```python
from build123d import *

# Parameters (mm, degrees)
RESSALTO_EXTRUS_O1_DEPTH = 150


with BuildPart() as part:
    # Esboço1 → Ressalto-extrusão1 (new body)
    with BuildSketch(Plane(origin=(0, 0, 0), x_dir=(1, 0, 0), z_dir=(0, 1, 0))):
        Polygon((3, 7.5), (7.5, 7.5), (7.5, -7.5), (7.5, -12.5047377), (2.5, -12.5047377), (2.5, -10.5847377), (4, -10.5847377), (4, -11.566741313), (6, -11.566741313), (6, -9.036092961), (-6, -9.036092961), (-6, -11.5647377), (-4, -11.5647377), (-4, -10.585059624), (-2.5, -10.585059624), (-2.5, -12.5047377), (-7.5, -12.5047377), (-7.5, -7.5), (-7.5, 7.5), (-3, 7.5), (-3, -2.5), (3, -2.5), align=None)
    extrude(amount=RESSALTO_EXTRUS_O1_DEPTH)


solid = part.part
```
CAD build for the part. Positions are in the model's coordinates, mm. A direction names the side the tool comes from. Coordinates: 2 decimals unless noted, no trailing zeros. Loops run counter-clockwise (first coordinate to the right, second up) from the corner with the lowest first, then second, coordinate; pieces in that order, holes last. Notation, with made-up numbers: (22, 25.5) - (73, 25.5) arc R27 cw to (73, 60.5) - close; hole circle Ø2 at (-11.5, 25.5). An arc over 180 degrees is marked (long way). Return JSON: item names as keys, results as strings.
1. Drop flat-ended pins along their axis: pin 1 (4 mm diameter, centred on x = -5.5, z = 10, fed in from -Y); pin 2 (1.5 mm diameter, centred on x = -1, y = 96.5, fed in from +Z). Give the stop position or say it passes through.
Result:
{"pin 1": "stops at y = 0", "pin 2": "stops at z = 9.04"}
2. Probe L1, parallel to X at y = 126, z = 11.5; L2, parallel to X at y = 24.5, z = -3; L3, parallel to Z at x = 3.25, y = 81.5. List the from-to ranges inside material, lowest first. Write a range as from..to.
Result:
{"L1": "x = -7.5..-6, -4..-2.5, 2.5..4, 6..7.5", "L2": "x = -7.5..-3, 3..7.5", "L3": "z = -7.5..9.04, 10.58..12.5"}
3. Mould opens along Z. For faces 4 (the flat face through (0, 150, 5)), 5 (the flat face through (6, 74, 10)), 6 (the flat face through (5, 74, -7.5)), 7 (the flat face through (-6, 74, 10)) say: released by +Z, released by -Z, zero draft, split by the parting line, or undercut.
Result:
{"face 4": "zero draft", "face 5": "undercut", "face 6": "released by -Z", "face 7": "undercut"}
4. Band-saw the part on A-A (z = -4). Give the cut face in (x, y).
Result:
{"outline": "(-7.5, 0) - (-3, 0) - (-3, 150) - (-7.5, 150) - close; (3, 0) - (7.5, 0) - (7.5, 150) - (3, 150) - close"}
5. 3-axis set-ups, long thin cutter, end or side, ignore diameter. For faces 1 (the flat face through (0, 74, 9.036)), 2 (the flat face through (-3, 74, -3)), 3 (the flat face through (-7.5, 74, 2)): which of +Z, -Z, +X, -X, +Y, -Y reach the whole face in a straight line?
Result:
{"face 1": "+Y, -Y", "face 2": "-Z, +Y, -Y", "face 3": "+Z, -Z, -X, +Y, -Y"}
6. Band-saw the part on B-B (y = 17.5). Give the cut face in (x, z).
Result:
{"outline": "(-7.5, -7.5) - (-3, -7.5) - (-3, 2.5) - (3, 2.5) - (3, -7.5) - (7.5, -7.5) - (7.5, 12.5) - (2.5, 12.5) - (2.5, 10.58) - (4, 10.58) - (4, 11.57) - (6, 11.57) - (6, 9.04) - (-6, 9.04) - (-6, 11.56) - (-4, 11.56) - (-4, 10.59) - (-2.5, 10.59) - (-2.5, 12.5) - (-7.5, 12.5) - close"}
